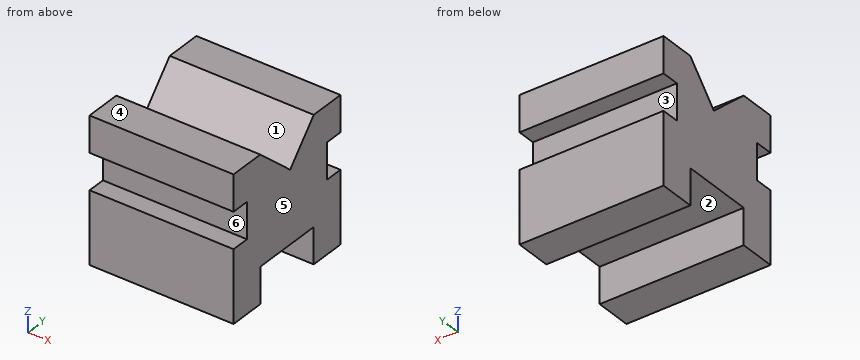
```python
from build123d import *

# Parameters (mm, degrees)
F0_W     = 101.6
F0_H     = 101.6
F1_DEPTH = 101.6
F2_W     = 12.7
F2_H     = 25.4
F3_DEPTH = 101.6
F4_W     = 50.8
F4_H     = 25.4
F5_DEPTH = 127
F6_W     = 12.7
F6_H     = 25.4
F7_DEPTH = 101.6
F9_DEPTH = 1397


with BuildPart() as f1:
    # F0 (on Front) → F1 (new body)
    with BuildSketch(Plane.XZ):
        with Locations((-50.8, 50.8)):
            Rectangle(F0_W, F0_H)
    extrude(amount=F1_DEPTH)

    # F2 (on face) → F3 (cut)
    with BuildSketch(Plane.YZ):
        with Locations((-95.25, 63.5)):
            Rectangle(F2_W, F2_H)
    extrude(amount=-F3_DEPTH, mode=Mode.SUBTRACT)

    # F4 (on face) → F5 (cut)
    with BuildSketch(Plane.YZ):
        with Locations((-50.8, 12.7)):
            Rectangle(F4_W, F4_H)
    extrude(amount=-F5_DEPTH, mode=Mode.SUBTRACT)

    # F6 (on face) → F7 (cut)
    with BuildSketch(Plane(origin=(-101.6, 0, 0), x_dir=(0, -1, 0), z_dir=(-1, 0, 0))):
        with Locations((6.35, 63.5)):
            Rectangle(F6_W, F6_H)
    extrude(amount=-F7_DEPTH, mode=Mode.SUBTRACT)

    # F8 (on face) → F9 (cut)
    with BuildSketch(Plane.YZ):
        Polygon((-25.4, 101.6), (-76.2, 101.6), (-47.801937, 76.2), align=None)
    extrude(amount=-F9_DEPTH, mode=Mode.SUBTRACT)


solid = f1.part
```
The model under review builds one solid part; all positions refer to its coordinate system, in mm. Face numbers are marked on the shaded views. A direction names the side the tool comes from. Coordinates: 2 decimals unless noted, no trailing zeros. Write each loop counter-clockwise with the first axis right and the second up, starting at its lowest first coordinate (ties: lowest second). Pieces come first, ordered by that corner, then holes. Notation, with made-up numbers: (32, 23.25) -> (73, 23.25) arc R29 cw to (73, 59.25) -> close; hole circle Ø6 at (-16.75, -32). An arc over 180 degrees is marked (long way). One line per item, written item: value. Start each with the question number.
Q1. Add section C-C, the plane z = 95. Give the boundary of the cut face in (x, y), then the cut area to 3 significant figures.
Q2. For the marked faces 1, 2 and 3, list the 3-axis set-ups (+Z, -Z, +X, -X, +Y, -Y) from which the entire face can be reached by the end or side of a thin tool; tool diameter is ignored.
Q3. Add section D-D, the plane z = 62.5. Give the boundary of the cut face in (x, y), then the cut area to 3 significant figures.
Q4. To check wall thickness, follow probe 1 along Y at (x, z) = (-18, 20); probe 2 along Z at (x, y) = (-42.5, -6); probe 3 along Y at (x, z) = (-29.5, 86). State the ranges of each line that lie inside material, in increasing order.
Q5. Add section B-B, the plane x = -29. Give the boundary of the cut face in (y, z), then the cut area to 3 significant figures.
Q6. The part is to be moulded in two halves that separate along Z. For the marked faces 4, 5 and 6, say which applies: +Z half, -Z half, draft (parallel to the pull), parting line (faces both ways), or undercut.
Q7. Clearance check with flat-ended pins moving along their axes: P1, Ø1, axis at x = -16, y = -63, coming from the -Z side; P2, Ø8, axis at x = -61, y = -48, coming from the +Z side. State where each tip first meets the part, or that it passes through.
Q8. Add section A-A, the plane z = 9.5. Give the boundary of the cut face in (x, y).
Response:
1. outline: (-101.6, -101.6) -> (0, -101.6) -> (0, -68.82) -> (-101.6, -68.82) -> close; (-101.6, -31.22) -> (0, -31.22) -> (0, 0) -> (-101.6, 0) -> close
1. area: 6,500 mm²
2. face 1: +Z, +X, -X
2. face 2: -Z, +X, -X
2. face 3: +X, -X, +Y
3. outline: (-101.6, -88.9) -> (0, -88.9) -> (0, -12.7) -> (-101.6, -12.7) -> close
3. area: 7,740 mm²
4. probe 1: -101.6 to -76.2, -25.4 to 0
4. probe 2: 0 to 50.8, 76.2 to 101.6
4. probe 3: -101.6 to -58.76, -39.16 to 0
5. outline: (-101.6, 0) -> (-76.2, 0) -> (-76.2, 25.4) -> (-25.4, 25.4) -> (-25.4, 0) -> (0, 0) -> (0, 50.8) -> (-12.7, 50.8) -> (-12.7, 76.2) -> (0, 76.2) -> (0, 101.6) -> (-25.4, 101.6) -> (-47.8, 76.2) -> (-76.2, 101.6) -> (-101.6, 101.6) -> (-101.6, 76.2) -> (-88.9, 76.2) -> (-88.9, 50.8) -> (-101.6, 50.8) -> close
5. area: 7,740 mm²
6. face 4: +Z half
6. face 5: draft
6. face 6: undercut
7. P1: z = 25.4
7. P2: z = 80.51
8. outline: (-101.6, -101.6) -> (0, -101.6) -> (0, -76.2) -> (-101.6, -76.2) -> close; (-101.6, -25.4) -> (0, -25.4) -> (0, 0) -> (-101.6, 0) -> close
